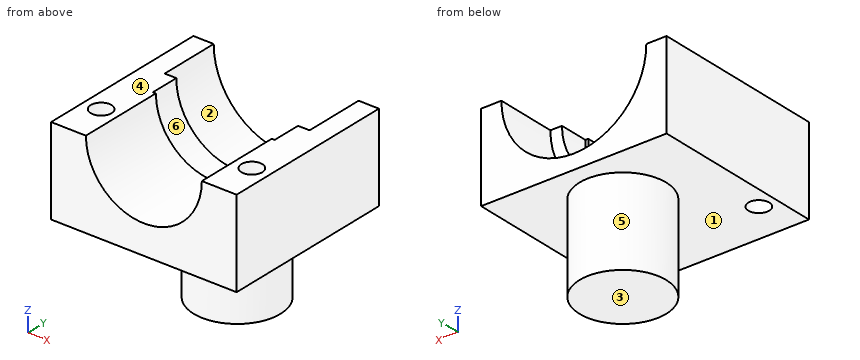
Autodesk Inventor part; units mm, degrees
ref_plane "YZ Plane" through (0, 0, 0) normal (1, 0, 0) x (0, 1, 0)
ref_plane "XZ Plane" through (0, 0, 0) normal (0, 1, 0) x (-1, 0, 0)
ref_plane "XY Plane" through (0, 0, 0) normal (0, 0, 1) x (1, 0, 0)
sketch "Skizze1" plane through (0, 0, 0) normal (0, 0, 1) x (1, 0, 0)
  line L0 (-16, 20) -> (16, 20)
  line L1 (16, 20) -> (16, -20)
  line L2 (16, -20) -> (-16, -20)
  line L3 (-16, -20) -> (-16, 20)
  line L4 (-16, 20) -> (16, -20) construction
  line L5 (16, 20) -> (-16, -20) construction
  point P0 (0, 0)
  dimension "d0" = 32
  dimension "d1" = 40
extrude "Extrusion1" add sketch "Skizze1" along normal blind 15
sketch "Skizze2" plane through (-16, -20, 0) normal (0, -1, 0) x (1, 0, 0)
  line L0 (0, 15) -> (32, 15)
  line L1 (0, 0) -> (0, 15)
  line L2 (32, 0) -> (0, 0)
  line L3 (32, 0) -> (32, 15)
  line L4 (32, 15) -> (0, 15)
  circle A0 centre (16, 15) radius 10
  point P0 (16, 0)
  dimension "d4" = 20
extrude "Extrusion2" cut sketch "Skizze2" against normal blind 15 contours A0 L0 | L0 A0
sketch "Skizze3" plane through (-16, -5, 0) normal (0, -1, 0) x (1, 0, 0)
  line L0 (0, 0) -> (0, 15)
  line L1 (32, 0) -> (0, 0)
  line L2 (32, 0) -> (32, 15)
  line L3 (26, 15) -> (32, 15)
  line L4 (0, 15) -> (6, 15)
  line L5 (6, 15) -> (26, 15)
  circle A0 centre (16, 15) radius 10.5
  point P0 (16, 0)
  dimension "d7" = 21
extrude "Extrusion3" cut sketch "Skizze3" against normal blind 5 contours A0 L3 L5 L4 | L4 L5 L3 A0
sketch "Skizze4" plane through (-16, 0, 0) normal (0, -1, 0) x (1, 0, 0)
  line L0 (5.5, 15) -> (26.5, 15)
  circle A0 centre (16, 15) radius 12.5
  point P0 (16, 0)
  dimension "d10" = 25
extrude "Extrusion4" cut sketch "Skizze4" against normal through all
sketch "Skizze5" plane through (0, 0, 15) normal (0, 0, 1) x (1, 0, 0)
  line L0 (-16, 20) -> (-16, -20)
  line L1 (-16, -20) -> (-10, -20)
  line L2 (-10, -20) -> (-10, -5)
  line L3 (10, -5) -> (10, -20)
  line L4 (10, -20) -> (16, -20)
  line L5 (16, -20) -> (16, 20)
  circle A0 centre (-13, -13) radius 1.8
  circle A1 centre (13, -13) radius 1.8
  point P0 (0, 0)
  dimension "d13" = 3.6
  dimension "d14" = 3.6
  dimension "d15" = 7
  dimension "d16" = 7
  dimension "d17" = 3
  dimension "d18" = 3
extrude "Extrusion5" cut sketch "Skizze5" against normal through all
sketch "Skizze8" plane through (0, 0, 0) normal (0, 0, -1) x (-1, 0, 0)
  line L0 (12.5, 20) -> (16, 20)
  line L1 (16, 20) -> (16, 10.5)
  line L2 (16, 20) -> (16, -20)
  line L3 (16, 10.5) -> (-16, 10.5)
  line L4 (-16, 20) -> (-16, -20)
  line L5 (16, 20) -> (-16, 20)
  line L6 (-16, 20) -> (16, 20)
  point P0 (0, 0)
  dimension "d28" = 9.5
extrude "Extrusion8" cut sketch "Skizze8" along normal mid plane 58.75
sketch "Skizze9" plane through (0, 0, 0) normal (0, 0, -1) x (-1, 0, 0)
  circle A0 centre (0, 0) radius 7.475
  dimension "d31" = 14.95
extrude "Extrusion9" add sketch "Skizze9" along normal blind 15
properties part number "5 Objektivhalterung unten"
Build history of the part. All positions in model axes, mm. Face numbers are marked on the shaded views. A direction names the side the tool comes from. Coordinates: 2 decimals unless noted, no trailing zeros. Order: outer loops, then holes, each group sorted by start corner. A loop starts at its lowest first (then second) coordinate and runs counter-clockwise, first axis right, second up. Notation, with made-up numbers: (55, 8.5) - (86, 8.5) arc R22 ccw to (86, 46.5) - close; hole circle Ø9 at (44.5, 32). An arc over 180 degrees is marked (long way). Write each question's results on one line, items separated by ' | '. Start each with the question number.
Item 1: Tool access for the marked faces 1, 2 and 3: list every direction of +Z, -Z, +X, -X, +Y, -Y with a clear straight run to the whole face (end or side of a thin tool).
Item 2: Band-saw the part on B-B on z = 6.75. Write the cut outline in (x, y).
Item 3: Band-saw the part on D-D on z = 0.75. Write the cut outline in (x, y), and give its area (3 significant figures).
Item 4: Band-saw the part on C-C on y = -8.5. Write the cut outline in (x, z), and give its area (3 significant figures).
Item 5: Wall check: probe 1 along Y at (x, z) = (13, 7); probe 2 along Z at (x, y) = (-15, 9); probe 3 along X at (y, z) = (-9, 12.5). Give the ranges that are in metal, low to high. Write a range as [from, to].
Item 6: Flat gauge pins, fed straight in: pin 1 (11.5 mm diameter, centred on x = -0.5, z = 10.5, fed in from +Y); pin 2 (6 mm diameter, centred on x = -7.5, y = -9.5, fed in from -Z); pin 3 (4.5 mm diameter, centred on x = -13, y = -13, fed in from +Z); pin 4 (4 mm diameter, centred on x = 2.5, z = -9.5, fed in from -Y). Where does each tip first touch, or does it go through?
Item 7: Mould opens along X. For the marked faces 4, 5 and 6 say: released by +X, released by -X, zero draft, split by the parting line, or undercut.
Item 8: Band-saw the part on A-A on x = 13. Write the cut outline in (y, z).
Numbers:
1) face 1: -Z | face 2: +Z, +Y | face 3: -Z, +X, -X, +Y, -Y
2) outline: (-16, -20) - (-5.65, -20) - (-5.65, -5) - (-6.5, -5) - (-6.5, 0) - (-9.39, 0) - (-9.39, 10.5) - (-16, 10.5) - close; (5.65, -20) - (16, -20) - (16, 10.5) - (9.39, 10.5) - (9.39, 0) - (6.5, 0) - (6.5, -5) - (5.65, -5) - close; hole circle Ø3.6 at (-13, -13); hole circle Ø3.6 at (13, -13)
3) outline: (-16, -20) - (16, -20) - (16, 10.5) - (-16, 10.5) - close; hole circle Ø3.6 at (-13, -13); hole circle Ø3.6 at (13, -13) | area: 956 mm^2
4) outline: (-16, 0) - (16, 0) - (16, 15) - (10, 15) arc R10 cw to (-10, 15) - (-16, 15) - close | area: 323 mm^2
5) probe 1: [-20, -14.8], [-11.2, 10.5] | probe 2: [0, 15] | probe 3: [-16, -9.68], [9.68, 16]
6) pin 1: y = -5 | pin 2: z = 0 | pin 3: z = 15 | pin 4: y = -7.46
7) face 4: zero draft | face 5: split by the parting line | face 6: undercut
8) outline: (-20, 0) - (-14.8, 0) - (-14.8, 15) - (-20, 15) - close; (-11.2, 0) - (10.5, 0) - (10.5, 15) - (-11.2, 15) - close
